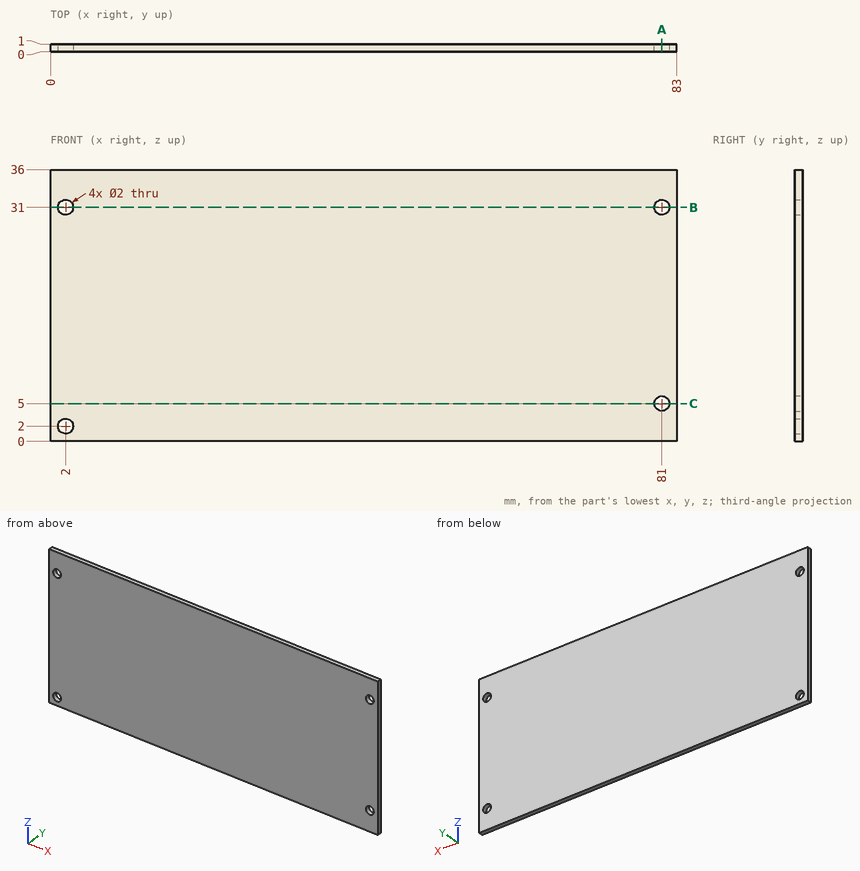
Study the drawing (mm; zero at the part's minimum x, y, z) and answer. Give positions to 0.01 mm unless a question says otherwise; leave off trailing zeros. Loops run counter-clockwise (first coordinate to the right, second up) from the corner with the lowest first, then second, coordinate; pieces in that order, holes last. Notation, with made-up numbers: (30.25, -5) - (46.25, -5) arc R24 cw to (46.25, 19) - close; hole circle Ø4 at (27.5, -10.75). An arc over 180 degrees is marked (long way). Return JSON: item names as keys, results as strings. Group by question number.
1. Straight lines are drawn through the part: line 1 (Z direction, x = 81, y = 0.3); line 2 (Z direction, x = 2, y = 0.45); line 3 (X direction, y = 0.4, z = 31). For each, find the intervals that lie inside material, in ascending order. Write a range as [from, to].
2. Find section A-A (x = 81). Write down the section's boundary in (y, z).
3. Given pin 1 Ø1.6 at (x, z) = (2, 31) entering from -Y, flat-ended and moving along its own axis, determine where the tip first touches the part or whether it passes through.
4. Find section B-B (z = 31). Write down the section's boundary in (x, y).
5. Find section C-C (z = 5). Write down the section's boundary in (x, y), then the cut area to 3 significant figures.
Verdict:
{
 "1": {"line 1": "z = [0, 4], [6, 30], [32, 36]", "line 2": "z = [0, 1], [3, 30], [32, 36]", "line 3": "x = [0, 1], [3, 80], [82, 83]"},
 "2": {"outline": "(0, 0) - (1, 0) - (1, 4) - (0, 4) - close; (0, 6) - (1, 6) - (1, 30) - (0, 30) - close; (0, 32) - (1, 32) - (1, 36) - (0, 36) - close"},
 "3": {"pin 1": "passes through"},
 "4": {"outline": "(0, 0) - (1, 0) - (1, 1) - (0, 1) - close; (3, 0) - (80, 0) - (80, 1) - (3, 1) - close; (82, 0) - (83, 0) - (83, 1) - (82, 1) - close"},
 "5": {"outline": "(0, 0) - (80, 0) - (80, 1) - (0, 1) - close; (82, 0) - (83, 0) - (83, 1) - (82, 1) - close", "area": "81.0 mm^2"}
}
